from build123d import *

# Parameters (mm, degrees)
SKETCH1_R           = 19
BOSS_EXTRUDE1_DEPTH = 8
FILLET1_R           = 0.5
SKETCH3_R           = 1.55
CUT_EXTRUDE1_DEPTH  = 8
SKETCH4_R           = 6.58897104
CUT_EXTRUDE2_DEPTH  = 8
CIRPATTERN1_COUNT   = 4


with BuildPart() as part:
    # Sketch1 → Boss-Extrude1 (new body)
    with BuildSketch(Plane.XY):
        Circle(SKETCH1_R)
    extrude(amount=BOSS_EXTRUDE1_DEPTH)

    # Sketch2 → Cut-Revolve1 (revolve, cut)
    with BuildSketch(Plane(origin=(0, 0, 0), x_dir=(0, 0, -1), z_dir=(1, 0, 0))):
        with BuildLine():
            Line((-7, 19), (-4.535200691, 19))
            ThreePointArc((-4.535200691, 19), (-5.767600345, 18.5), (-7, 19))
        make_face()
        with BuildLine():
            Line((-3.535200691, 19), (-1, 19))
            ThreePointArc((-1, 19), (-2.267600345, 18.7), (-3.535200691, 19))
        make_face()
    revolve(axis=Axis((0, 0, 8.4), (0, 0, -1)), mode=Mode.SUBTRACT)

    # Fillet1
    fillet1_edges = [part.edges().sort_by_distance(p)[0] for p in [
        (-19, 0, 0),
        (-19, 0, 8),
    ]]
    fillet(fillet1_edges, radius=FILLET1_R)

    # Sketch3 → Cut-Extrude1 (cut)
    with BuildSketch(Plane.XY.offset(8)):
        Circle(SKETCH3_R)
    extrude(amount=-CUT_EXTRUDE1_DEPTH, mode=Mode.SUBTRACT)

    # Sketch4 → Cut-Extrude2 (cut)
    with BuildSketch(Plane.XY.offset(8)):
        with Locations((0, 10.60646011)):
            Circle(SKETCH4_R)
    cut_extrude2 = extrude(amount=-CUT_EXTRUDE2_DEPTH, mode=Mode.SUBTRACT)

    # CirPattern1: Cut-Extrude2 ×4 about axis
    cirpattern1_axis = Axis((0, 0, 0), (0, 0, 1))
    for i in range(1, CIRPATTERN1_COUNT):
        add(cut_extrude2.rotate(cirpattern1_axis, i * 360 / CIRPATTERN1_COUNT), mode=Mode.SUBTRACT)


solid = part.part
Input: part model. Units: mm. Frame: model coordinates. Round coordinates to 2 decimals unless told otherwise and drop trailing zeros. Order: outer loops, then holes, each group sorted by start corner. A loop starts at its lowest first (then second) coordinate and runs counter-clockwise, first axis right, second up. Notation, with made-up numbers: (35.25, 19) - (40.25, 19) arc R21 ccw to (40.25, 27) - close; hole circle Ø6 at (62.5, 45.5). An arc over 180 degrees is marked (long way). Answer as a JSON object with one key per item and string values. Group by question number.
(1) Cut plane A-A (y = 0). Return loops of the section in (x, z).
(2) Cut plane D-D (z = 6). Return loops of the section in (x, y).
(3) Pin query (flat end, axial travel): P1, Ø21, axis at x = 0, y = 10.61, coming from the -Z side; P2, Ø3, axis at y = -14, z = 4.5, coming from the -X side; P3, Ø1.5, axis at x = -7.5, z = 6, coming from the -Y side. Return the tip coordinate at first contact, or that it passes through.
(4) Cut plane C-C (z = 2). Return loops of the section in (x, y).
(5) Draft query along X for faces 1 (the face through (18.12, 5.71, 4.03)), 2 (the face through (0.86, -17.14, 4.06)), 3 (the face through (-0.26, -3.85, 0)). Return one class per face: released by +X, released by -X, zero draft, split by the parting line, or undercut.
(6) Material intervals for probe 1 along X at (y, z) = (-3, 5.5); probe 2 along X at (y, z) = (-5.5, 5); probe 3 along Y at (x, z) = (-5.5, 1), sorted ascending. Write a range as from..to.
Here are the results:
{
 "1": {"outline": "(-19, 0.5) arc R0.5 ccw to (-18.5, 0) - (-17.2, 0) - (-17.2, 8) - (-18.5, 8) arc R0.5 ccw to (-19, 7.5) - (-19, 7) arc R1.77 cw to (-19, 4.54) - (-19, 3.54) arc R2.83 cw to (-19, 1) - close; (-4.02, 0) - (-1.55, 0) - (-1.55, 8) - (-4.02, 8) - close; (1.55, 0) - (4.02, 0) - (4.02, 8) - (1.55, 8) - close; (17.2, 0) - (18.5, 0) arc R0.5 ccw to (19, 0.5) - (19, 1) arc R2.83 cw to (19, 3.54) - (19, 4.54) arc R1.77 cw to (19, 7) - (19, 7.5) arc R0.5 ccw to (18.5, 8) - (17.2, 8) - close"},
 "2": {"outline": "circle Ø37.03 at (0, 0); hole circle Ø13.18 at (-10.61, 0); hole circle Ø13.18 at (0, -10.61); hole circle Ø13.18 at (0, 10.61); hole circle Ø3.1 at (0, 0); hole circle Ø13.18 at (10.61, 0)"},
 "3": {"P1": "stops at z = 0", "P2": "stops at x = -14.31", "P3": "stops at y = -17.33"},
 "4": {"outline": "circle Ø37.43 at (0, 0); hole circle Ø13.18 at (-10.61, 0); hole circle Ø13.18 at (0, -10.61); hole circle Ø13.18 at (0, 10.61); hole circle Ø3.1 at (0, 0); hole circle Ø13.18 at (10.61, 0)"},
 "5": {"face 1": "split by the parting line", "face 2": "undercut", "face 3": "zero draft"},
 "6": {"probe 1": "x = -18.28..-16.47, -4.74..4.74, 16.47..18.28", "probe 2": "x = -17.85..-14.23, -6.98..-4.16, 4.16..6.98, 14.23..17.85", "probe 3": "y = -18.19..-14.23, -6.98..-4.16, 4.16..6.98, 14.23..18.19"}
}
